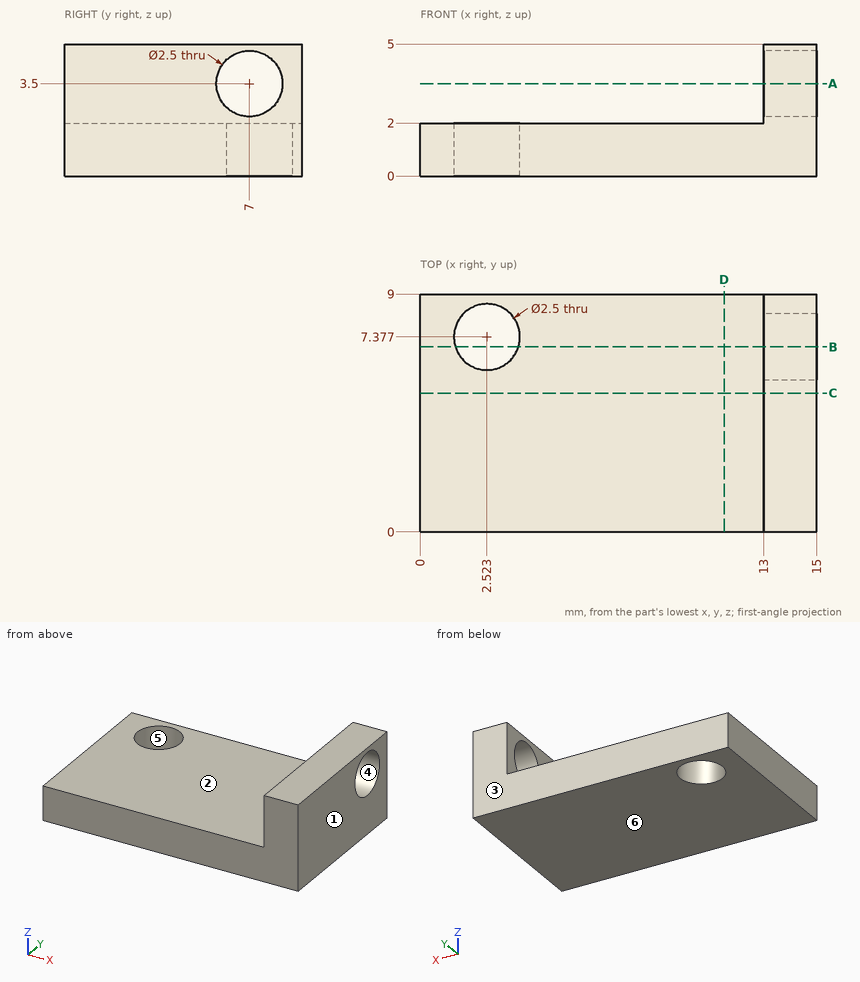
Here's the drawing with two shaded views (mm, measured from the low corner). I have some questions. A direction names the side the tool comes from. Round coordinates to 2 decimals unless told otherwise and drop trailing zeros. Loops run counter-clockwise (first coordinate to the right, second up) from the corner with the lowest first, then second, coordinate; pieces in that order, holes last. Notation, with made-up numbers: (31, -22.5) - (58, -22.5) arc R10 ccw to (58, -7.5) - close; hole circle Ø3 at (-1, 4.25). An arc over 180 degrees is marked (long way). Write item = value, one per line.
1) I need wall thicknesses on line 1 along Z through (x, y) = (13.55, 7); line 2 along Z through (x, y) = (5.5, 4.25); line 3 along X through (y, z) = (2.75, 4.2). Which ranges of each line are inside material? Lowest first, please. Write a range as from..to.
Computed:
line_1 = 0..2.25, 4.75..5
line_2 = 0..2
line_3 = 13..15
2) Imagine slicing it at A-A (z = 3.5). Please give me the cut outline in (x, y).
Computed:
outline = (13, 0) - (15, 0) - (15, 5.75) - (13, 5.75) - close; (13, 8.25) - (15, 8.25) - (15, 9) - (13, 9) - close
3) Imagine slicing it at B-B (y = 7). Give the number of separate pieces and of enclosed holes in the cut face.
Computed:
separate_pieces = 3
enclosed_holes = 0
4) Imagine slicing it at C-C (y = 5.25). Please give me the cut outline in (x, z).
Computed:
outline = (0, 0) - (15, 0) - (15, 5) - (13, 5) - (13, 2) - (0, 2) - close
5) I'm going to push flat-ended pins straight in: P1, Ø4.5, axis at x = 9, y = 3, coming from the +Z side; P2, Ø1, axis at x = 6, y = 8, coming from the -Z side. Where does each tip first touch, or does it pass through?
Computed:
P1 = 2
P2 = 0
6) Imagine slicing it at D-D (x = 11.5). Please give me the cut outline in (y, z).
Computed:
outline = (0, 0) - (9, 0) - (9, 2) - (0, 2) - close
7) If we mould it in two halves opening along Y, with no side actions, what happens to the marked faces 3, 4, 5 and 6? For each: pulls with the +Y half, pulls with the -Y half, needs draft (parallel to the pull), parting line crosses it, or undercut.
Computed:
face_3 = pulls with the +Y half
face_4 = undercut
face_5 = undercut
face_6 = needs draft
8) On a 3-axis mill with a long thin cutter (end or side, diameter ignored), from which of +Z, -Z, +X, -X, +Y, -Y can I reach the whole of each face in a straight line? I mean the marked faces 1 and 2. Say none if no direction works.
Computed:
face_1 = +Z, -Z, +X, +Y, -Y
face_2 = +Z, -X, +Y, -Y
